Can you work these out from the drawing? Everything is in mm from the part's minimum corner. A direction names the side the tool comes from. Round coordinates to 2 decimals unless told otherwise and drop trailing zeros. Loops run counter-clockwise (first coordinate to the right, second up) from the corner with the lowest first, then second, coordinate; pieces in that order, holes last. Notation, with made-up numbers: (-14, 60.25) - (40, 60.25) arc R20 ccw to (40, 88.25) - close; hole circle Ø9 at (-36.75, -10). An arc over 180 degrees is marked (long way). Answer as a JSON object with one key per item and string values. Group by question number.
1) I want a section at C-C, the plane x = 60. Please give me the cut outline in (y, z), then the cut area to 3 significant figures.
2) I want a section at A-A, the plane z = 20. Please give me the cut outline in (x, y).
3) I want a section at B-B, the plane x = 25. Please give me the cut outline in (y, z), then the cut area to 3 significant figures.
4) Will these pins go through, and if not, where does the flat tip stop? P1, Ø1, axis at y = 3.5, z = 10.5, coming from the -X side; P2, Ø6, axis at x = 36.5, z = 21, coming from the -Y side; P3, Ø2, axis at y = 2.5, z = 10.5, coming from the -X side; P4, Ø1.5, axis at x = 27.5, y = 4.5, coming from the +Z side.
5) Which directions (+Z, -Z, +X, -X, +Y, -Y) give clear straight access to the entire face, cutting with the end or side of a thin tool? Please do the marked faces 4 and 5.
6) If we mould it in two halves opening along Z, with no side actions, what happens to the marked faces 1, 2 and 3? For each: pulls with the +Z half, pulls with the -Z half, needs draft (parallel to the pull), parting line crosses it, or undercut.
7) If I drill on line 1 along Z through (x, y) = (60, 4.65); line 2 along Z through (x, y) = (25, 2.55); line 3 along Z through (x, y) = (10.5, 1.7), over which ranges is the centre line in solid material (lowest first)? Write a range as [from, to].
8) I want a section at D-D, the plane y = 4.2. Please give me the cut outline in (x, z), then the cut area to 3 significant figures.
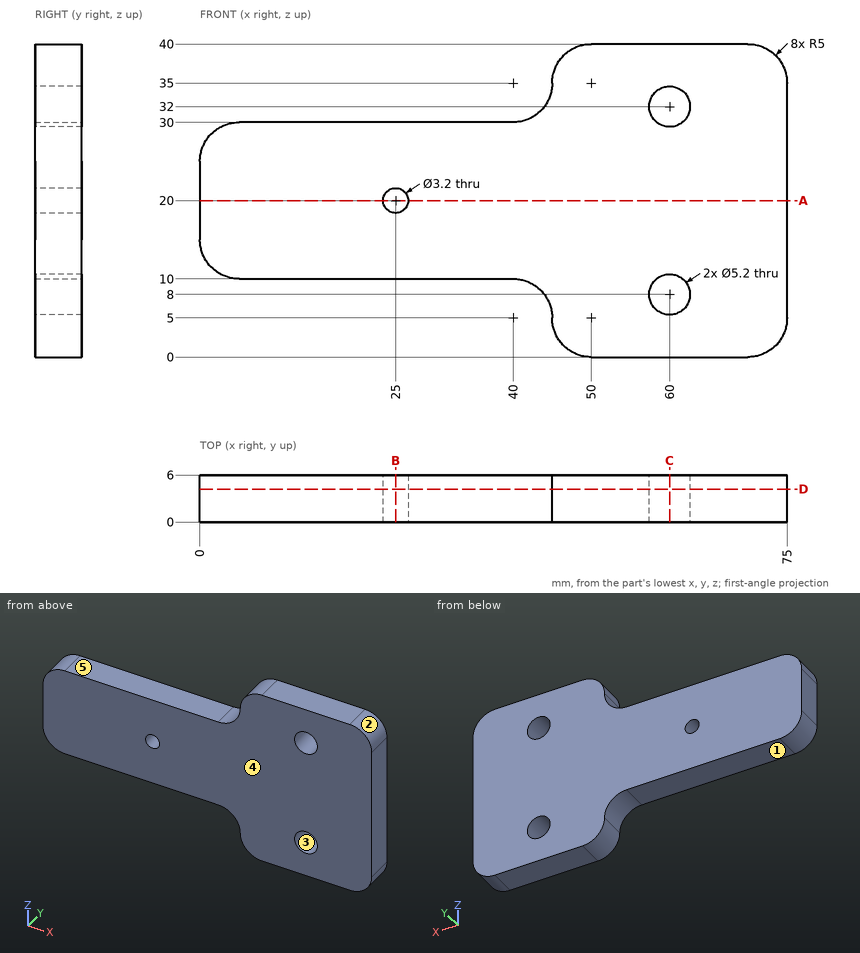
Outcome:
{
 "1": {"outline": "(0, 0) - (6, 0) - (6, 5.4) - (0, 5.4) - close; (0, 10.6) - (6, 10.6) - (6, 29.4) - (0, 29.4) - close; (0, 34.6) - (6, 34.6) - (6, 40) - (0, 40) - close", "area": "178 mm^2"},
 "2": {"outline": "(0, 0) - (23.4, 0) - (23.4, 6) - (0, 6) - close; (26.6, 0) - (75, 0) - (75, 6) - (26.6, 6) - close"},
 "3": {"outline": "(0, 10) - (6, 10) - (6, 18.4) - (0, 18.4) - close; (0, 21.6) - (6, 21.6) - (6, 30) - (0, 30) - close", "area": "101 mm^2"},
 "4": {"P1": "x = 2", "P2": "y = 0", "P3": "x = 1.43", "P4": "z = 30"},
 "5": {"face 4": "+Z, -Z, +X, -X, -Y", "face 5": "+Z, -X, +Y, -Y"},
 "6": {"face 1": "pulls with the -Z half", "face 2": "pulls with the +Z half", "face 3": "undercut"},
 "7": {"line 1": "[0, 5.4], [10.6, 29.4], [34.6, 40]", "line 2": "[10, 18.4], [21.6, 30]", "line 3": "[10, 30]"},
 "8": {"outline": "(0, 15) arc R5 ccw to (5, 10) - (40, 10) arc R5 cw to (45, 5) arc R5 ccw to (50, 0) - (70, 0) arc R5 ccw to (75, 5) - (75, 35) arc R5 ccw to (70, 40) - (50, 40) arc R5 ccw to (45, 35) arc R5 cw to (40, 30) - (5, 30) arc R5 ccw to (0, 25) - close; hole circle Ø3.2 at (25, 20); hole circle Ø5.2 at (60, 8); hole circle Ø5.2 at (60, 32)", "area": "2,030 mm^2"}
}
